from build123d import *

# Parameters (mm, degrees)
SKETCH2_W                   = 1390
SKETCH2_H                   = 1000
SKETCH2_W_2                 = 1265
SKETCH2_H_2                 = 875
BOSS_EXTRUDE1_DEPTH         = 534.5
SKETCH3_W                   = 1390
SKETCH3_H                   = 1000
BOSS_EXTRUDE2_DEPTH         = 62.5
MMRTG_START                 = -62.5
MMRTG_HOLDER_DEPTH          = 5
SKETCH5_R                   = 12.5
SUSPENSION_BOLT_HOLES_DEPTH = 1571.920192117
CONTROL_ARM_CUTOUT_REACH    = 1331.931
SKETCH6_W                   = 50
SKETCH6_H                   = 225
MIRROR3_COPY_1_REACH        = 1331.931
MIRROR3_COPY_1_SKETCH_W     = 50
MIRROR3_COPY_1_SKETCH_H     = 225
SKETCH7_W                   = 1515
SKETCH7_H                   = 1105
SKETCH7_W_2                 = 1265
SKETCH7_H_2                 = 875
ATTACHROVERFLANGE_DEPTH     = 10
SKETCH11_R                  = 12.5
BOSS_EXTRUDE3_DEPTH         = 5
SKETCH13_R                  = 25
SKETCH13_W                  = 15
SKETCH13_H                  = 300
BOSS_EXTRUDE4_DEPTH         = 250
CUT_EXTRUDE1_DEPTH          = 250
CUT_EXTRUDE1_DEPTH_BACK     = 15
SKETCH14_W                  = 400
SKETCH14_H                  = 55.53291541
CUT_EXTRUDE2_REACH          = 1269.282
SKETCH15_R                  = 5
SKETCH16_W                  = 400
SKETCH16_H                  = 66.742444313
CUT_EXTRUDE3_DEPTH          = 607


with BuildPart() as part:
    # Sketch2 → Boss-Extrude1 (new body)
    with BuildSketch(Plane(origin=(0, 0, 0), x_dir=(1, 0, 0), z_dir=(0, 1, 0))):
        Rectangle(SKETCH2_W, SKETCH2_H)
        Rectangle(SKETCH2_W_2, SKETCH2_H_2, mode=Mode.SUBTRACT)
    extrude(amount=-BOSS_EXTRUDE1_DEPTH)

    # Sketch3 → Boss-Extrude2 (add)
    with BuildSketch(Plane.XZ.offset(534.5)):
        Rectangle(SKETCH3_W, SKETCH3_H)
    extrude(amount=-BOSS_EXTRUDE2_DEPTH)

    # Sketch4 → MMRTG Holder (add)
    with BuildSketch(Plane(origin=(695, 0, 0), x_dir=(0, 0, -1), z_dir=(1, 0, 0)).offset(MMRTG_START)):
        with BuildLine():
            Line((-105, -261), (-110, -261))
            ThreePointArc((-110, -261), (0, -371), (110, -261))
            Line((110, -261), (105, -261))
            ThreePointArc((105, -261), (0, -366), (-105, -261))
        make_face()
    mmrtg_holder = extrude(amount=-MMRTG_HOLDER_DEPTH)

    # Mirror1: MMRTG Holder across plane
    add(mmrtg_holder.mirror(Plane(origin=(0, 0, 0), x_dir=(0, 0, 1), z_dir=(1, 0, 0))))

    # Sketch5 → Suspension Bolt Holes (cut, through all)
    with BuildSketch(Plane(origin=(695, 0, 0), x_dir=(0, 0, -1), z_dir=(1, 0, 0))):
        with Locations((-400, -309.5)):
            Circle(SKETCH5_R)
        with Locations((-400, -434.5)):
            Circle(SKETCH5_R)
        with Locations((400, -434.5)):
            Circle(SKETCH5_R)
        with Locations((400, -309.5)):
            Circle(SKETCH5_R)
    extrude(amount=-SUSPENSION_BOLT_HOLES_DEPTH, mode=Mode.SUBTRACT)

    # Sketch6 → Control Arm Cutout (cut, up to next)
    with BuildSketch(Plane(origin=(0, 0, -500), x_dir=(-1, 0, 0), z_dir=(0, 0, -1)), mode=Mode.PRIVATE) as control_arm_cutout_sk1:
        with Locations((-607.5, -359.5)):
            Rectangle(SKETCH6_W, SKETCH6_H)
    control_arm_cutout_tool1 = extrude(control_arm_cutout_sk1.sketch, amount=-CONTROL_ARM_CUTOUT_REACH, mode=Mode.PRIVATE) & part.part
    control_arm_cutout = control_arm_cutout_tool1.solids().sort_by_distance((607.5, -359.5, -500))[0]
    add(control_arm_cutout, mode=Mode.SUBTRACT)

    # Mirror2: Control Arm Cutout across plane
    add(control_arm_cutout.mirror(Plane(origin=(0, 0, 0), x_dir=(0, 0, 1), z_dir=(1, 0, 0))), mode=Mode.SUBTRACT)

    # Mirror3: Control Arm Cutout across plane
    add(control_arm_cutout.mirror(Plane.XY), mode=Mode.SUBTRACT)

    # Mirror3 copy 1 sketch → Mirror3 copy 1 (cut, up to next)
    with BuildSketch(Plane.XY.offset(500), mode=Mode.PRIVATE) as mirror3_copy_1_sk1:
        with Locations((-607.5, -359.5)):
            Rectangle(MIRROR3_COPY_1_SKETCH_W, MIRROR3_COPY_1_SKETCH_H)
    mirror3_copy_1_tool1 = extrude(mirror3_copy_1_sk1.sketch, amount=-MIRROR3_COPY_1_REACH, mode=Mode.PRIVATE) & part.part
    add(mirror3_copy_1_tool1.solids().sort_by_distance((-607.5, -359.5, 500))[0], mode=Mode.SUBTRACT)

    # Sketch7 → AttachRoverFlange (add)
    with BuildSketch(Plane(origin=(0, 0, 0), x_dir=(1, 0, 0), z_dir=(0, 1, 0))):
        Rectangle(SKETCH7_W, SKETCH7_H)
        Rectangle(SKETCH7_W_2, SKETCH7_H_2, mode=Mode.SUBTRACT)
    extrude(amount=-ATTACHROVERFLANGE_DEPTH)

    # Sketch11 → Boss-Extrude3 (add)
    with BuildSketch(Plane(origin=(695, 0, 0), x_dir=(0, 0, -1), z_dir=(1, 0, 0))):
        with Locations((-400, -309.5)):
            Circle(SKETCH11_R)
        with Locations((-400, -434.5)):
            Circle(SKETCH11_R)
        with Locations((400, -309.5)):
            Circle(SKETCH11_R)
        with Locations((400, -434.5)):
            Circle(SKETCH11_R)
    boss_extrude3 = extrude(amount=-BOSS_EXTRUDE3_DEPTH)

    # Mirror4: Boss-Extrude3 across plane
    add(boss_extrude3.mirror(Plane(origin=(0, 0, 0), x_dir=(0, 0, 1), z_dir=(1, 0, 0))))

    # Sketch13 → Boss-Extrude4 (add, symmetric)
    with BuildSketch(Plane(origin=(0, 0, 0), x_dir=(0, 0, -1), z_dir=(1, 0, 0))):
        with Locations((507.5, -134.5)):
            Circle(SKETCH13_R)
        with Locations((507.5, -284.5)):
            Rectangle(SKETCH13_W, SKETCH13_H)
    boss_extrude4 = extrude(amount=BOSS_EXTRUDE4_DEPTH, both=True)

    # Sketch14 → Cut-Extrude1 (cut, two sides: drawn at the far end of the back side and taken through both)
    with BuildSketch(Plane(origin=(0, 0, -515), x_dir=(-1, 0, 0), z_dir=(0, 0, -1)).offset(-CUT_EXTRUDE1_DEPTH_BACK)):
        with Locations((0, -130.58202233)):
            Rectangle(SKETCH14_W, SKETCH14_H)
    extrude(amount=CUT_EXTRUDE1_DEPTH + CUT_EXTRUDE1_DEPTH_BACK, mode=Mode.SUBTRACT)

    # Cut-Extrude2: up to this face of the body (flat: up to its plane)
    cut_extrude2_end = Plane(part.part.faces().sort_by_distance((-695, -272.25, 0))[0])
    # Sketch15 → Cut-Extrude2 (cut, up to the picked face)
    with BuildSketch(Plane(origin=(250, 0, 0), x_dir=(0, 0, -1), z_dir=(1, 0, 0)), mode=Mode.PRIVATE) as cut_extrude2_sk1:
        with Locations((515, -132.090441405)):
            Circle(SKETCH15_R)
    cut_extrude2_tool1 = split(extrude(cut_extrude2_sk1.sketch, amount=-CUT_EXTRUDE2_REACH, mode=Mode.PRIVATE), bisect_by=cut_extrude2_end, keep=Keep.BOTH, mode=Mode.PRIVATE)
    cut_extrude2 = cut_extrude2_tool1.solids().sort_by(Axis((250, -132.090441, -515), (-1, 0, 0)))[0]
    add(cut_extrude2, mode=Mode.SUBTRACT)

    # Mirror6: Boss-Extrude4, Cut-Extrude2 across plane
    add(boss_extrude4.mirror(Plane.XY))
    add(cut_extrude2.mirror(Plane.XY), mode=Mode.SUBTRACT)

    # Sketch16 → Cut-Extrude3 (cut)
    with BuildSketch(Plane.XY.offset(500)):
        with Locations((0, -124.977257879)):
            Rectangle(SKETCH16_W, SKETCH16_H)
    extrude(amount=CUT_EXTRUDE3_DEPTH, mode=Mode.SUBTRACT)


solid = part.part
Geometry: final body of the model. Coordinates: model frame, mm. A direction names the side the tool comes from. Coordinates: 2 decimals unless noted, no trailing zeros. Order: outer loops, then holes, each group sorted by start corner. A loop starts at its lowest first (then second) coordinate and runs counter-clockwise, first axis right, second up.
1) Draft query along Z for faces 1 (the cylindrical face through (630.035, -365.975, -2.309)), 2 (the flat face through (200, -134, 509)). Return one class per face: released by +Z, released by -Z, zero draft, split by the parting line, or undercut.
Result sheet:
face 1: undercut
face 2: zero draft
2) Section A-A (y = -214). Return loops of the section in (x, z), then the cut area to 3 significant figures.
Result sheet:
outline: (-695, -500) - (-250, -500) - (-250, -515) - (250, -515) - (250, -500) - (695, -500) - (695, 500) - (250, 500) - (250, 515) - (-250, 515) - (-250, 500) - (-695, 500) - close; hole (-632.5, -437.5) - (632.5, -437.5) - (632.5, 437.5) - (-632.5, 437.5) - close
area: 298,000 mm2
3) Section C-C (y = -78). Return loops of the section in (x, z), then the cut area to 3 significant figures.
Result sheet:
outline: (-695, -500) - (695, -500) - (695, 500) - (-695, 500) - close; hole (-632.5, -437.5) - (632.5, -437.5) - (632.5, 437.5) - (-632.5, 437.5) - close
area: 283,000 mm2
4) Ray query, probe 1 along Y at (x, z) = (-665, -400); probe 2 along X at (y, z) = (-251, 490); probe 3 along X at (y, z) = (-186, -99). Return the intervals inside material, ascending.
Result sheet:
probe 1: y = -534.5 to -447, -422 to -322, -297 to 0
probe 2: x = -695 to -632.5, -582.5 to 582.5, 632.5 to 695
probe 3: x = -695 to -632.5, 632.5 to 695
5) First-contact query: P1, Ø2, axis at x = -458, z = -267, coming from the +Y side; P2, Ø3, axis at y = -435.5, z = 320, coming from the +X side; P3, Ø10, axis at y = -283, z = -513.5, coming from the -X side; P4, Ø4, axis at x = -631, z = 106.5, coming from the +Y side. Flat tips, straight axial feed; report the tip coordinate or a pass-through.
Result sheet:
P1: stops at y = -472
P2: stops at x = 695
P3: stops at x = -250
P4: stops at y = 0
6) Set-up query: faces 3 (the flat face through (-608, -247, -469)), 4 (the flat face through (250, -270, 509)), 5 (the flat face through (-695, -269, 7)). Return all of +Z, -Z, +X, -X, +Y, -Y with unobstructed straight access to the full face (end or side cutting, diameter ignored); none if empty.
Result sheet:
face 3: +Z, -Z
face 4: +Z, +X, -Y
face 5: +Z, -Z, -X, -Y
7) Section D-D (z = -29). Return loops of the section in (x, y), then the cut area to 3 significant figures.
Result sheet:
outline: (-757.5, -10) - (-695, -10) - (-695, -534.5) - (695, -534.5) - (695, -10) - (757.5, -10) - (757.5, 0) - (632.5, 0) - (632.5, -361.92) - (627.5, -361.92) - (627.5, -367.11) - (632.5, -367.11) - (632.5, -472) - (-632.5, -472) - (-632.5, -367.11) - (-627.5, -367.11) - (-627.5, -361.92) - (-632.5, -361.92) - (-632.5, 0) - (-757.5, 0) - close
area: 147,000 mm2
8) Section B-B (x = -290). Return loops of the section in (y, z).
Result sheet:
outline: (-534.5, -500) - (-10, -500) - (-10, -552.5) - (0, -552.5) - (0, -437.5) - (-472, -437.5) - (-472, 437.5) - (0, 437.5) - (0, 552.5) - (-10, 552.5) - (-10, 500) - (-534.5, 500) - close
